```python
from build123d import *

# Parameters (mm, degrees)
SKETCH_1_R               = 16.5
DIAMETER33_HEIGHT8_DEPTH = 8
CHARACTER_DEPTH          = 0.1
SKETCH_3_R               = 13.1
SKETCH_3_R_2             = 12.7
INK_RING_DEPTH           = 0.08


with BuildPart() as part:
    # 草图1 → Diameter33_Height8 (new body)
    with BuildSketch(Plane.XY):
        Circle(SKETCH_1_R)
    extrude(amount=-DIAMETER33_HEIGHT8_DEPTH)

    # 草图2 → Character_马 (add)
    with BuildSketch(Plane.XY):
        with BuildLine():
            add(Edge.make_bspline(
                [(-2.543859649, 2.657894737), (-2.568109523, 2.601908638), (-2.618944351, 2.484545403), (-2.68091831, 2.29374228), (-2.747882739, 2.084905171), (-2.809197893, 1.853949883), (-2.867938942, 1.601351852), (-2.929388828, 1.329074257), (-2.981674213, 1.034530608), (-3.05538164, 0.620649676), (-3.127595616, 0.098084884), (-3.197623224, -0.517816396), (-3.237414282, -1.112851594), (-3.242919292, -1.502329954), (-3.245614035, -1.692982456)],
                knots=[0, 0, 0, 0, 0.495689669, 1.0391105, 1.629386371, 2.27856569, 2.980637221, 3.737641002, 4.547078417, 5.411969332, 7.15491927, 8.834024839, 10.450232028, 12, 12, 12, 12], degree=3))
            Line((-3.245614035, -1.692982456), (2.50877193, -1.692982456))
            add(Edge.make_bspline(
                [(2.50877193, -1.692982456), (2.555842668, -1.219109546), (2.651092154, -0.26020911), (2.765765857, 0.939059138), (2.857689962, 1.892225125), (2.928191701, 2.576627854), (2.997770846, 3.225611417), (3.046502797, 3.646446892), (3.070175439, 3.850877193)],
                knots=[0, 0, 0, 0, 1.538264342, 3.112738277, 3.891618687, 4.631513556, 5.335226919, 6, 6, 6, 6], degree=3))
            Line((3.070175439, 3.850877193), (-3.666666667, 3.850877193))
            add(Edge.make_bspline(
                [(-3.666666667, 3.850877193), (-3.893660384, 3.849684604), (-4.355478431, 3.847258285), (-5.06158577, 3.833290973), (-5.793776141, 3.813732), (-6.290908298, 3.791840575), (-6.543859649, 3.780701754)],
                knots=[0, 0, 0, 0, 0.946376728, 1.925400653, 2.944399995, 4, 4, 4, 4], degree=3))
            Line((-6.543859649, 3.780701754), (-6.543859649, 5.184210526))
            add(Edge.make_bspline(
                [(-6.543859649, 5.184210526), (-6.290908298, 5.173071706), (-5.793776141, 5.15118028), (-5.06158577, 5.131621308), (-4.355478431, 5.117653996), (-3.893660384, 5.115227677), (-3.666666667, 5.114035088)],
                knots=[0, 0, 0, 0, 1.055600005, 2.074599347, 3.053623272, 4, 4, 4, 4], degree=3))
            Line((-3.666666667, 5.114035088), (4.684210526, 5.114035088))
            add(Edge.make_bspline(
                [(4.684210526, 5.114035088), (4.594389665, 4.480170947), (4.4139847, 3.207056477), (4.243054526, 1.774416685), (4.14478495, 0.828967937), (4.097381465, 0.388144624), (4.055421695, -0.025950303), (4.020061293, -0.412530658), (3.985399458, -0.77104386), (3.956533585, -1.101987754), (3.933708028, -1.406199086), (3.919206962, -1.600281379), (3.912280702, -1.692982456)],
                knots=[0, 0, 0, 0, 2.802935976, 5.629689589, 6.316260642, 6.964711014, 7.570877404, 8.13855511, 8.664335647, 9.147876972, 9.592993668, 10, 10, 10, 10], degree=3))
            Line((3.912280702, -1.692982456), (7.140350877, -1.692982456))
            add(Edge.make_bspline(
                [(7.140350877, -1.692982456), (7.117496771, -1.957195671), (7.070752869, -2.497595555), (7.005207646, -3.329223298), (6.94597212, -4.200007765), (6.901683429, -4.946124678), (6.868307152, -5.546229635), (6.826684596, -5.980862849), (6.785382047, -6.39647152), (6.728695376, -6.792040318), (6.670245675, -7.168463089), (6.603590191, -7.526033406), (6.524025139, -7.862448123), (6.444320105, -8.179786345), (6.348007699, -8.470700422), (6.240664659, -8.735979197), (6.112879912, -8.969541099), (5.972363355, -9.176368475), (5.813514, -9.350805736), (5.639780874, -9.496502029), (5.450674708, -9.612389616), (5.239809272, -9.700393942), (4.996758723, -9.765827824), (4.713795659, -9.832208089), (4.381558555, -9.885783366), (4.002176073, -9.941267696), (3.574948301, -9.992657478), (3.098313267, -10.039000074), (2.574062445, -10.080415008), (2.208184758, -10.1025182), (2.01754386, -10.114035088)],
                knots=[0, 0, 0, 0, 1.887044686, 3.859605311, 5.935782741, 8.09729868, 9.178245636, 10.211890598, 11.203790184, 12.149721099, 13.054774096, 13.914409008, 14.736879022, 15.514410289, 16.241554355, 16.915874949, 17.547596075, 18.132428342, 18.691003543, 19.220627564, 19.740803274, 20.262911441, 20.840419939, 21.529816771, 22.330465222, 23.233668769, 24.258284961, 25.391864306, 26.641028549, 28, 28, 28, 28], degree=3))
            add(Edge.make_bspline(
                [(2.01754386, -10.114035088), (1.999634211, -9.981554353), (1.962380573, -9.705982807), (1.828075725, -9.291338106), (1.637078715, -8.859880402), (1.472081327, -8.577306965), (1.385964912, -8.429824561)],
                knots=[0, 0, 0, 0, 0.882983811, 1.83668375, 2.870909156, 4, 4, 4, 4], degree=3))
            add(Edge.make_bspline(
                [(1.385964912, -8.429824561), (1.601684871, -8.434299725), (2.00798008, -8.44272842), (2.580650352, -8.452457271), (3.078902343, -8.449896251), (3.50262546, -8.439476904), (3.851072115, -8.425325844), (4.125715661, -8.404487351), (4.325845969, -8.373466937), (4.498441923, -8.324930212), (4.647964297, -8.219854178), (4.806608465, -8.080366), (4.946574967, -7.900402806), (5.057213348, -7.72659571), (5.135709742, -7.551771137), (5.19099419, -7.380870408), (5.241966461, -7.171945715), (5.293801136, -6.927772939), (5.340465741, -6.64505285), (5.379651802, -6.325610866), (5.42315596, -5.969892033), (5.467875091, -5.457573461), (5.519200344, -4.8262348), (5.563244909, -4.113096685), (5.591709685, -3.474461181), (5.594963512, -3.073991037), (5.596491228, -2.885964912)],
                knots=[0, 0, 0, 0, 1.758141494, 3.31135083, 4.666771348, 5.817797705, 6.764703246, 7.508656711, 8.059921999, 8.414932624, 8.957450007, 9.527295967, 10.134772448, 10.806750365, 11.201697625, 11.692819884, 12.268105713, 12.953448137, 13.726378385, 14.601998413, 15.575707604, 16.646246692, 18.791940105, 20.736977137, 22.467966827, 24, 24, 24, 24], degree=3))
            Line((5.596491228, -2.885964912), (-4.789473684, -2.885964912))
            add(Edge.make_bspline(
                [(-4.789473684, -2.885964912), (-4.742500482, -2.409482331), (-4.646861986, -1.439353083), (-4.506084048, 0.025074391), (-4.381186338, 1.489718928), (-4.325531367, 2.461946264), (-4.298245614, 2.938596491)],
                knots=[0, 0, 0, 0, 0.982838397, 2.001081075, 3.019997563, 4, 4, 4, 4], degree=3))
            add(Edge.make_bspline(
                [(-4.298245614, 2.938596491), (-4.000143593, 2.892268938), (-3.414928922, 2.801321673), (-2.830558232, 2.705101429), (-2.543859649, 2.657894737)],
                knots=[0, 0, 0, 0, 1.018778359, 2, 2, 2, 2], degree=3))
        make_face()
        with BuildLine():
            add(Edge.make_bspline(
                [(1.175438596, -5.061403509), (1.272474939, -5.06183074), (1.474359506, -5.062719598), (1.787949201, -5.055481089), (2.124128563, -5.051460824), (2.48108109, -5.043574331), (2.860490404, -5.031942174), (3.261734399, -5.023647615), (3.685265265, -5.005984943), (3.974652272, -4.996224852), (4.122807018, -4.99122807)],
                knots=[0, 0, 0, 0, 0.789853886, 1.643294733, 2.553146486, 3.526589248, 4.549556957, 5.643022245, 6.793320254, 8, 8, 8, 8], degree=3))
            Line((4.122807018, -4.99122807), (4.122807018, -6.324561404))
            add(Edge.make_bspline(
                [(4.122807018, -6.324561404), (3.969453719, -6.319579397), (3.671400907, -6.309896522), (3.237471852, -6.292228161), (2.829302521, -6.283816356), (2.447289567, -6.272341119), (2.09207297, -6.264362463), (1.762823851, -6.260344735), (1.460498309, -6.253100348), (1.267276772, -6.253971776), (1.175438596, -6.254385965)],
                knots=[0, 0, 0, 0, 1.248975298, 2.427470434, 3.535041912, 4.572114753, 5.538512415, 6.427215019, 7.252455469, 8, 8, 8, 8], degree=3))
            Line((1.175438596, -6.254385965), (-5.070175439, -6.254385965))
            add(Edge.make_bspline(
                [(-5.070175439, -6.254385965), (-5.298037146, -6.255493864), (-5.742534486, -6.257655079), (-6.391477007, -6.271227092), (-7.005930309, -6.290151347), (-7.403331701, -6.313306629), (-7.596491228, -6.324561404)],
                knots=[0, 0, 0, 0, 1.081761786, 2.110228356, 3.081464224, 4, 4, 4, 4], degree=3))
            Line((-7.596491228, -6.324561404), (-7.596491228, -4.99122807))
            add(Edge.make_bspline(
                [(-7.596491228, -4.99122807), (-7.403331701, -5.002482845), (-7.005930309, -5.025638127), (-6.391477007, -5.044562382), (-5.742534486, -5.058134395), (-5.298037146, -5.06029561), (-5.070175439, -5.061403509)],
                knots=[0, 0, 0, 0, 0.918535776, 1.889771644, 2.918238214, 4, 4, 4, 4], degree=3))
            Line((-5.070175439, -5.061403509), (1.175438596, -5.061403509))
        make_face()
    extrude(amount=CHARACTER_DEPTH)

    # 草图3 → Ink_ring (add)
    with BuildSketch(Plane.XY):
        with Locations(Location((0, 0, 0), (0, 0, 180))):
            Circle(SKETCH_3_R)
        with Locations(Location((0, 0, 0), (0, 0, 180))):
            Circle(SKETCH_3_R_2, mode=Mode.SUBTRACT)
    extrude(amount=INK_RING_DEPTH)


solid = part.part
```
Design review of the part built by this model. Coordinates are the model's own, in mm. A direction names the side the tool comes from. Round coordinates to 2 decimals unless told otherwise and drop trailing zeros. Write each loop counter-clockwise with the first axis right and the second up, starting at its lowest first coordinate (ties: lowest second). Pieces come first, ordered by that corner, then holes.
Item 1: We need section D-D on x = -11.5. Write out the cut boundary in (y, z), and give its area (3 significant figures).
Item 2: The part is to be moulded in two halves that separate along Y. For faces 3 (the cylindrical face through (15.24, -6.32, -3.94)), 4 (the flat face through (2, -2, 0.1)), 5 (the flat face through (0, 0, 0)), say which applies: +Y half, -Y half, draft (parallel to the pull), parting line (faces both ways), or undercut.
Item 3: We need section A-A on y = 10. Write out the cut boundary in (x, z), and give its area (3 significant figures).
Item 4: We need section C-C on z = -7.25. Write out the cut boundary in (x, y), and give its area (3 significant figures).
Item 5: Clearance check with flat-ended pins moving along their axes: pin 1 Ø2 at (x, z) = (9.5, -6.5) entering from +Y; pin 2 Ø1 at (y, z) = (-11.5, -4.5) entering from -X; pin 3 Ø4 at (x, z) = (-5, -3.5) entering from -Y (3 decimals). State where each tip first meets the part, or that it passes through.
Item 6: For probe 1 along Z at (x, y) = (-12.5, -3.5); probe 2 along Z at (x, y) = (1, 8); probe 3 along X at (y, z) = (0.5, -2.75), list the stretches that pass through material, from the lowest coordinate up.
Item 7: We need section B-B on x = -2. Write out the cut boundary in (y, z), and give its area (3 significant figures).
Item 8: For faces 1 (the flat face through (-2, -6, 0.1)), 2 (the flat face through (-10, 9, 0)), list the 3-axis set-ups (+Z, -Z, +X, -X, +Y, -Y) from which the entire face can be reached by the end or side of a thin tool; tool diameter is ignored.
Returned:
1. outline: (-11.83, -8) - (11.83, -8) - (11.83, 0) - (6.27, 0) - (6.27, 0.08) - (5.39, 0.08) - (5.39, 0) - (-5.39, 0) - (-5.39, 0.08) - (-6.27, 0.08) - (-6.27, 0) - (-11.83, 0) - close
1. area: 189 mm2
2. face 3: parting line
2. face 4: draft
2. face 5: undercut
3. outline: (-13.12, -8) - (13.12, -8) - (13.12, 0) - (8.46, 0) - (8.46, 0.08) - (7.83, 0.08) - (7.83, 0) - (-7.83, 0) - (-7.83, 0.08) - (-8.46, 0.08) - (-8.46, 0) - (-13.12, 0) - close
3. area: 210 mm2
4. outline: circle Ø33 at (0, 0)
4. area: 855 mm2
5. pin 1: stops at y = 14.14
5. pin 2: stops at x = -12.3
5. pin 3: stops at y = -16.225
6. probe 1: z = -8 to 0.08
6. probe 2: z = -8 to 0
6. probe 3: x = -16.49 to 16.49
7. outline: (-16.38, -8) - (16.38, -8) - (16.38, 0) - (12.95, 0) - (12.95, 0.08) - (12.54, 0.08) - (12.54, 0) - (5.11, 0) - (5.11, 0.1) - (3.85, 0.1) - (3.85, 0) - (-1.69, 0) - (-1.69, 0.1) - (-2.89, 0.1) - (-2.89, 0) - (-5.06, 0) - (-5.06, 0.1) - (-6.25, 0.1) - (-6.25, 0) - (-12.54, 0) - (-12.54, 0.08) - (-12.95, 0.08) - (-12.95, 0) - (-16.38, 0) - close
7. area: 262 mm2
8. face 1: +Z, +X, -X, +Y, -Y
8. face 2: +Z
